from build123d import *

# Parameters (mm, degrees)
F0_R      = 15
F0_R_2    = 4
F1_DEPTH  = 10
F2_R      = 15
F2_R_2    = 5
F3_DEPTH  = 30
F4_R      = 0.3
F5_R      = 0.3
F6_R      = 2
F7_DEPTH  = 20.34312
F9_DEPTH  = 10
F11_DEPTH = 10


with BuildPart() as f1:
    # F0 (on Top) → F1 (new body)
    with BuildSketch(Plane.XY):
        Circle(F0_R)
        Circle(F0_R_2, mode=Mode.SUBTRACT)
    extrude(amount=F1_DEPTH)

    # F2 (on face) → F3 (join)
    with BuildSketch(Plane.XY.offset(10)):
        Circle(F2_R)
        Circle(F2_R_2, mode=Mode.SUBTRACT)
    extrude(amount=F3_DEPTH)

    # F4
    f4_edges = [f1.edges().sort_by_distance(p)[0] for p in [
        (-15, 0, 40),
    ]]
    fillet(f4_edges, radius=F4_R)

    # F5
    f5_edges = [f1.edges().sort_by_distance(p)[0] for p in [
        (-15, 0, 0),
        (-5, 0, 40),
        (-4, 0, 0),
    ]]
    fillet(f5_edges, radius=F5_R)

    # F6 (on Front) → F7 (cut)
    with BuildSketch(Plane.XZ):
        with Locations((9, 34.7)):
            Circle(F6_R)
        with Locations((-9, 5.3)):
            Circle(F6_R)
    extrude(amount=-F7_DEPTH, mode=Mode.SUBTRACT)

    # F8 (on face) → F9 (cut)
    with BuildSketch(Plane.XY.offset(40)):
        with BuildLine():
            Line((2.5762253208, -0.1799123052), (5.2969454936, -0.1799123052))
            ThreePointArc((5.2969454936, -0.1799123052), (5.2992363184, -0.0899691164), (5.3, 0))
            ThreePointArc((5.3, 0), (5.2992363184, 0.0899691164), (5.2969454936, 0.1799123052))
            Line((5.2969454936, 0.1799123052), (2.5762253208, 0.1799123052))
            Line((2.5762253208, 0.1799123052), (2.5762253208, -0.1799123052))
        make_face()
        with BuildLine():
            Line((5.2969454936, -0.1799123052), (14.6988989915, -0.1799123052))
            ThreePointArc((14.6988989915, -0.1799123053), (14.6997247453, -0.0899578371), (14.7, 0))
            ThreePointArc((14.7, 0), (14.6997247453, 0.0899578371), (14.6988989915, 0.1799123053))
            Line((14.6988989915, 0.1799123052), (5.2969454936, 0.1799123052))
            ThreePointArc((5.2969454936, 0.1799123052), (5.2992363184, 0.0899691164), (5.3, 0))
            ThreePointArc((5.3, 0), (5.2992363184, -0.0899691164), (5.2969454936, -0.1799123052))
        make_face()
        with BuildLine():
            Line((14.6988989915, -0.1799123052), (17.0045065461, -0.1799123052))
            Line((17.0045065461, -0.1799123052), (17.0045065461, 0.1799123052))
            Line((17.0045065461, 0.1799123052), (14.6988989915, 0.1799123052))
            ThreePointArc((14.6988989915, 0.1799123053), (14.6997247453, 0.0899578371), (14.7, 0))
            ThreePointArc((14.7, 0), (14.6997247453, -0.0899578371), (14.6988989915, -0.1799123053))
        make_face()
    extrude(amount=-F9_DEPTH, mode=Mode.SUBTRACT)

    # F10 (on face) → F11 (cut)
    with BuildSketch(Plane(origin=(0, 0, 0), x_dir=(1, 0, 0), z_dir=(0, 0, -1))):
        with BuildLine():
            Line((-4.2962360163, -0.1798779937), (-1.9751195796, -0.1798779937))
            Line((-1.9751195796, -0.1798779937), (-1.9751195796, 0.1799466168))
            Line((-1.9751195796, 0.1799466168), (-4.2962331425, 0.1799466168))
            ThreePointArc((-4.2962331425, 0.1799466168), (-4.2999999999, 3.43417e-05), (-4.2962360163, -0.1798779937))
        make_face()
        with BuildLine():
            Line((-14.6988994114, -0.1798779937), (-4.2962360163, -0.1798779937))
            ThreePointArc((-4.2962360163, -0.1798779937), (-4.2999999999, 3.43417e-05), (-4.2962331425, 0.1799466168))
            Line((-4.2962331425, 0.1799466168), (-14.6988985715, 0.1799466168))
            ThreePointArc((-14.6988985715, 0.1799466168), (-14.7, 3.43142e-05), (-14.6988994114, -0.1798779937))
        make_face()
        with BuildLine():
            Line((-16.4034008048, -0.1798779937), (-14.6988994114, -0.1798779937))
            ThreePointArc((-14.6988994114, -0.1798779937), (-14.7, 3.43142e-05), (-14.6988985715, 0.1799466168))
            Line((-14.6988985715, 0.1799466168), (-16.4034008048, 0.1799466168))
            Line((-16.4034008048, 0.1799466168), (-16.4034008048, -0.1798779937))
        make_face()
    extrude(amount=-F11_DEPTH, mode=Mode.SUBTRACT)


solid = f1.part
Input: part model. Units: mm. Frame: model coordinates. A direction names the side the tool comes from. Give positions to 0.01 mm unless a question says otherwise; leave off trailing zeros. Order: outer loops, then holes, each group sorted by start corner. A loop starts at its lowest first (then second) coordinate and runs counter-clockwise, first axis right, second up. Notation, with made-up numbers: (50, -24) - (102, -24) arc R14 cw to (102, -10) - close; hole circle Ø8 at (-35.5, 88.25). An arc over 180 degrees is marked (long way). Answer as a JSON object with one key per item and string values. Group by question number.
Q1. Cut plane A-A, the plane x = 0. Output: boundary loops of the cut face in (y, z).
Q2. Mould query, pull axis X, two halves, no side actions, for faces 4 (the face through (-11, 0.18, 4)), 5 (the face through (-1.08, -4.88, 24.64)), 6 (the face through (7.002, 6.632, 34.788)), 7 (the face through (-14.985, 0.66, 19.724)). Classes: pulls with the +X half, pulls with the -X half, needs draft (parallel to the pull), parting line crosses it, or undercut.
Q3. Cut plane C-C, the plane z = 38. Output: boundary loops of the cut face in (x, y).
Q4. Line query: probe 1 along Z at (x, y) = (9, 10); probe 2 along X at (y, z) = (3, 14); probe 3 along Y at (x, z) = (0, 17.5). Output: solid intervals per line, ascending.
Q5. Cut plane D-D, the plane z = 24.5. Output: boundary loops of the cut face in (x, y), then the cut area to 3 significant figures.
Q6. Cut plane B-B, the plane z = 5.3. Output: boundary loops of the cut face in (x, y), then the cut area to 3 significant figures.
Q7. Set-up query: faces 1 (the face through (-4, 2, 10)), 2 (the face through (-9, -0.18, 5)), 3 (the face through (-7.153, 6.632, 4.534)). Return all of +Z, -Z, +X, -X, +Y, -Y with unobstructed straight access to the full face (end or side cutting, diameter ignored); none if empty.
Q8. First-contact query: pin 1 Ø8 at (x, z) = (-8.5, 7) entering from -Y; pin 2 Ø3 at (x, z) = (-7, 4.5) entering from +Y; pin 3 Ø8 at (x, z) = (9, 37.5) entering from -Y. Flat tips, straight axial feed; report the tip coordinate or a pass-through.
Results:
{
 "1": {"outline": "(-15, 0.3) arc R0.3 ccw to (-14.7, 0) - (-4.3, 0) arc R0.3 ccw to (-4, 0.3) - (-4, 10) - (-5, 10) - (-5, 39.7) arc R0.3 ccw to (-5.3, 40) - (-14.7, 40) arc R0.3 ccw to (-15, 39.7) - close; (4, 0.3) arc R0.3 ccw to (4.3, 0) - (14.7, 0) arc R0.3 ccw to (15, 0.3) - (15, 39.7) arc R0.3 ccw to (14.7, 40) - (5.3, 40) arc R0.3 ccw to (5, 39.7) - (5, 10) - (4, 10) - close"},
 "2": {"face 4": "needs draft", "face 5": "undercut", "face 6": "undercut", "face 7": "parting line crosses it"},
 "3": {"outline": "(5, -0.18) arc R5 cw (long way) to (5, 0.18) - (15, 0.18) arc R15 ccw (long way) to (15, -0.18) - close"},
 "4": {"probe 1": "0 to 32.7, 36.7 to 40", "probe 2": "-14.7 to -4, 4 to 14.7", "probe 3": "-15 to -5, 5 to 15"},
 "5": {"outline": "circle Ø30 at (0, 0); hole circle Ø10 at (0, 0)", "area": "628 mm^2"},
 "6": {"outline": "(-15, -0.18) arc R15 ccw (long way) to (-7, 13.27) - (-7, 0.18) - (-4, 0.18) arc R4 cw (long way) to (-4, -0.18) - close; (-15, 0.18) - (-11, 0.18) - (-11, 10.2) arc R15 ccw to start", "area": "606 mm^2"},
 "7": {"face 1": "+Z", "face 2": "-Z, -X", "face 3": "+Y"},
 "8": {"pin 1": "y = -14.31", "pin 2": "y = 13.96", "pin 3": "y = -14.14"}
}
